Build history of the part. All positions in model axes, mm. Give positions to 0.01 mm unless a question says otherwise; leave off trailing zeros. Loops run counter-clockwise (first coordinate to the right, second up) from the corner with the lowest first, then second, coordinate; pieces in that order, holes last. Notation, with made-up numbers: M -7.5,-10 L 27.5,-10 A23 cw 27.5,27 Z; hole C -27.75,-29 d4. An arc over 180 degrees is marked long. Put each result on its own line as item: value.
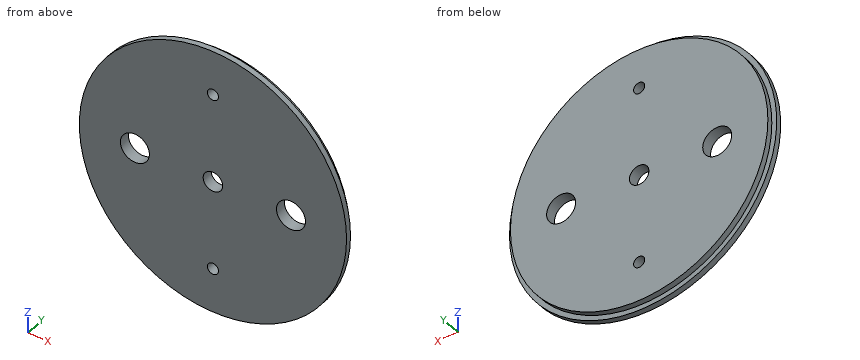
```python
from build123d import *

# Parameters (mm, degrees)
SKETCH1_R                   = 73.3171
SKETCH1_R_2                 = 76.0984
BOSS_EXTRUDE1_DEPTH         = 3.175
SKETCH1_3_R                 = 73.3171
BOSS_EXTRUDE2_DEPTH         = 6.35
F_1_4_0_25_DIAMETER_HOLE1_D = 6.35
M18X1_5_TAPPED_HOLE1_D      = 16.5
SKETCH3_3_R                 = 5.55625
CUT_EXTRUDE2_DEPTH          = 7.35


with BuildPart() as part:
    # Sketch1 → Boss-Extrude1 (new body)
    with BuildSketch(Plane(origin=(0, 0, 0), x_dir=(1, 0, 0), z_dir=(0, 1, 0))):
        Circle(SKETCH1_R)
        Circle(SKETCH1_R_2)
        Circle(SKETCH1_R, mode=Mode.SUBTRACT)
    extrude(amount=BOSS_EXTRUDE1_DEPTH)

    # Sketch1_3 → Boss-Extrude2 (add)
    with BuildSketch(Plane(origin=(0, 0, 0), x_dir=(1, 0, 0), z_dir=(0, 1, 0))):
        Circle(SKETCH1_3_R)
    extrude(amount=BOSS_EXTRUDE2_DEPTH)

    # 1_4 _0.25_ Diameter Hole1 (through all)
    with Locations(Plane(origin=(0, 0, 0), x_dir=(-1, 0, 0), z_dir=(0, -1, 0))):
        with Locations((0, 50.8), (0, -50.8)):
            Hole(F_1_4_0_25_DIAMETER_HOLE1_D / 2)

    # M18x1.5 Tapped Hole1 (through all)
    with Locations(Plane(origin=(0, 0, 0), x_dir=(-1, 0, 0), z_dir=(0, -1, 0))):
        with Locations((44.45, 0), (-44.45, 0)):
            Hole(M18X1_5_TAPPED_HOLE1_D / 2)

    # Sketch3_3 → Cut-Extrude2 (cut, through all)
    with BuildSketch(Plane.XZ):
        Circle(SKETCH3_3_R)
    extrude(amount=-CUT_EXTRUDE2_DEPTH, mode=Mode.SUBTRACT)


solid = part.part
```
Q1. Slice it at D-D (y = 1.25). State how many separate pieces and enclosed holes the cut face has, and give its area (3 significant figures).
Here are the results:
separate pieces: 1
enclosed holes: 5
area: 17,600 mm²
Q2. Drop flat-ended pins along their axis: pin 1 Ø3 at (y, z) = (3.5, -8.5) entering from +X; pin 2 Ø3 at (x, y) = (47, 4.5) entering from +Z. Give the stop position or say it passes through.
Here are the results:
pin 1: x = 75.77
pin 2: z = 60.4
Q3. Slice it at A-A (z = 0). List the corners of the cut face in (x, y) (3 decimals), and give its area (3 significant figures).
Here are the results:
outline: M -76.098,0 L -52.7,0 L -52.7,6.35 L -73.317,6.35 L -73.317,3.175 L -76.098,3.175 Z; M -36.2,0 L -5.556,0 L -5.556,6.35 L -36.2,6.35 Z; M 5.556,0 L 36.2,0 L 36.2,6.35 L 5.556,6.35 Z; M 52.7,0 L 76.098,0 L 76.098,3.175 L 73.317,3.175 L 73.317,6.35 L 52.7,6.35 Z
area: 669 mm²
Q4. Slice it at C-C (x = 45.5). List the corners of the cut face in (y, z) (3 decimals), and give its area (3 significant figures).
Here are the results:
outline: M 0,-60.998 L 3.175,-60.998 L 3.175,-57.49 L 6.35,-57.49 L 6.35,-8.183 L 0,-8.183 Z; M 0,8.183 L 6.35,8.183 L 6.35,57.49 L 3.175,57.49 L 3.175,60.998 L 0,60.998 Z
area: 648 mm²
Q5. Slice it at B-B (x = 0). List the corners of the cut face in (y, z) (3 decimals), and give its area (3 significant figures).
Here are the results:
outline: M 0,-76.098 L 3.175,-76.098 L 3.175,-73.317 L 6.35,-73.317 L 6.35,-53.975 L 0,-53.975 Z; M 0,-47.625 L 6.35,-47.625 L 6.35,-5.556 L 0,-5.556 Z; M 0,5.556 L 6.35,5.556 L 6.35,47.625 L 0,47.625 Z; M 0,53.975 L 6.35,53.975 L 6.35,73.317 L 3.175,73.317 L 3.175,76.098 L 0,76.098 Z
area: 798 mm²
Q6. Probe line 1 (Z direction, x = -0.5, y = 3.5); line 2 (Z direction, x = 0, y = 2) (3 decimals); line 3 (X direction, y = 1, z = 1). List the from-to ranges inside material, lowest first. Write a range as from..to.
Here are the results:
line 1: -73.32..-53.94, -47.66..-5.53, 5.53..47.66, 53.94..73.32
line 2: -76.098..-53.975, -47.625..-5.556, 5.556..47.625, 53.975..76.098
line 3: -76.09..-52.64, -36.26..-5.47, 5.47..36.26, 52.64..76.09
